CAD build for the part. Positions are in the model's coordinates, mm. Give positions to 0.01 mm unless a question says otherwise; leave off trailing zeros. Order: outer loops, then holes, each group sorted by start corner. A loop starts at its lowest first (then second) coordinate and runs counter-clockwise, first axis right, second up. Notation, with made-up numbers: (73.5, 21.25) -> (111.5, 21.25) arc R28 cw to (111.5, 45.25) -> close; hole circle Ø9 at (-14.5, 0). An arc over 180 degrees is marked (long way). Use one line per item in the form item = value. Start each with the question number.
1) Mould opens along Y. For faces 1 (the face through (0, 14, 0)), 2 (the face through (3.53, 55.87, 0.25)), 3 (the face through (-0.47, 0.67, 0.25)) say: pulls with the +Y half, pulls with the -Y half, needs draft (parallel to the pull), parting line crosses it, or undercut.
2) Cut at D-D, the plane x = -12. Give the cut face in (y, z).
3) Probe line 1 (X direction, y = 3, z = 0.4); line 2 (Y direction, x = 1, z = 0.15); line 3 (Y direction, x = 8, z = 0.4). List the from-to ranges inside material, lowest first.
4) Drop a flat-ended pin along its axis: P1, Ø3, axis at x = 7, y = -23.5, coming from the +Z side. Give the stop position or say it passes through.
5) Cut at C-C, the plane y = -21. Give the cut face in (x, z).
6) Cut at A-A, the plane x = 4. Give the cut face in (y, z), and give its area (3 significant figures).
7) Cut at B-B, the plane z = 0.35. Give the cut face in (x, y).
Autodesk Inventor part; units mm, degrees
ref_plane "YZ Plane" through (0, 0, 0) normal (1, 0, 0) x (0, 1, 0)
ref_plane "XZ Plane" through (0, 0, 0) normal (0, 1, 0) x (-1, 0, 0)
ref_plane "XY Plane" through (0, 0, 0) normal (0, 0, 1) x (1, 0, 0)
sketch "Sketch1" plane through (0, 0, 0) normal (0, 0, 1) x (1, 0, 0)
  line L0 (-17.5, -33.2499) -> (-17.5, 57.9837)
  arc A0 (-10.0449, 58.8745) -> (-17.5, 57.9837) centre (-12.5, 47.7794) ccw
  line L1 (-10.0449, 58.8745) -> (17.5, 52.7794)
  line L2 (17.5, 52.7794) -> (17.5, -15.7501)
  line L3 (17.5, -15.7501) -> (-17.5, -33.2499)
  line L4 (0.5, 7.1892) -> (0.5, 22.231)
  line L5 (0.5, 22.231) -> (-5.8925, 22.231)
  line L6 (-5.8925, 22.231) -> (-5.8925, 7.1892)
  line L7 (-5.8925, 7.1892) -> (0.5, 7.1892)
  point P0 (0, 0)
extrude "Extrusion1" add sketch "Sketch1" along normal blind 0.5 contours L0 A0 L1 L2 L3 | L7 L6 L5 L4
sketch "Sketch2" plane through (0, 0, 0.5) normal (0, 0, 1) x (1, 0, 0)
  line L0 (-1.5084, -24.1362) -> (-5.5333, -16.0863)
  line L1 (-5.5333, -16.0863) -> (-14.5107, -20.575)
  line L2 (-14.5107, -20.575) -> (-10.1014, -29.3938)
  arc A0 (-17.5, -30.0139) -> (-14.6056, -31.8027) centre (-15.5, -30.0139) ccw
  line L3 (-17.5, -30.0139) -> (-17.5, -1.8864)
  line L4 (-17.5, -1.8864) -> (-7.5, -1.8864)
  line L5 (-7.5, -1.8864) -> (-7.5, 7.5751)
  line L6 (-7.5, 7.5751) -> (-8.8, 7.5751)
  line L7 (-8.8, 26.3195) -> (-8.8, 7.5751)
  spline S0 degree 3 poles (-14.2046, 28.2052) (-13.4118, 28.2052) (-12.6544, 28.0226) (-10.9379, 27.4679) (-9.855, 26.8958) (-8.8077, 26.3237) (-8.8038, 26.3216) (-8.8, 26.3195) knots -0.001308 -0.001308 -0.001308 -0.001308 0.187612 0.187612 0.544343 0.544343 0.545651 0.545651 0.545651 0.545651
  line L8 (-14.2046, 28.2052) -> (-17.5, 28.2052)
  line L9 (-17.5, 28.2052) -> (-17.5, 31.9794)
  arc A1 (-17.5, 31.9794) -> (-4.376, 33.2499) centre (-12.5, 48.7499) ccw
  arc A2 (-4.376, 33.2499) -> (2.7674, 54.4137) centre (-12.5, 47.7794) ccw
  arc A3 (3.9006, 55.7887) -> (2.7674, 54.4137) centre (3.6845, 54.8123) ccw
  line L10 (3.9006, 55.7887) -> (16.7161, 52.9529)
  arc A4 (17.5, 51.9765) -> (16.7161, 52.9529) centre (16.5, 51.9765) ccw
  line L11 (-17.5, 57.9837) -> (-17.5, -33.2499)
  line L12 (-17.5, -33.2499) -> (17.5, -15.7501)
  line L13 (17.5, -15.7501) -> (17.5, 52.7794)
  line L14 (17.5, 52.7794) -> (-10.0449, 58.8745)
  arc A5 (-10.0449, 58.8745) -> (-17.5, 57.9837) centre (-12.5, 47.7794) ccw
  line L15 (5.1606, 7.0459) -> (-1.321, 3.6769)
  line L16 (4.7678, -6.2957) -> (11.3303, -6.2957)
  line L17 (11.3303, -6.2957) -> (11.3303, 7.0459)
  circle A6 centre (5.4296, 0.5354) radius 5.9007
  line L18 (5.4296, 0.5354) -> (11.3303, 0.5354)
  line L19 (11.3303, 0.5354) -> (11.3303, 6.4362)
  line L20 (11.3303, 6.4362) -> (5.4296, 6.4362)
  line L21 (5.4296, 6.4362) -> (5.4296, 0.5354)
  line L22 (11.3303, 0.5354) -> (5.4296, 0.5354)
  line L23 (5.4296, 0.5354) -> (5.4296, -5.3653)
  line L24 (5.4296, -5.3653) -> (11.3303, -5.3653)
  line L25 (11.3303, -5.3653) -> (11.3303, 0.5354)
  line L26 (17.5, 51.9765) -> (17.5, -14.6321)
  line L27 (17.5, -14.6321) -> (-1.4167, -24.7491)
  arc A7 (-1.4167, -24.7491) -> (-1.5084, -24.1362) centre (-2.4029, -24.5834) ccw
  line L28 (-10.1014, -29.3938) -> (-14.6056, -31.8027)
  point P0 (0, 0)
  point P1 (17.5, 7.0459)
  point P2 (17.5, -15.0638)
extrude "Extrusion2" cut sketch "Sketch2" against normal blind 10 contours L24 A6 L17 | A6 L20 L17 | L18 L21 A6 | A6 L23 L18 | A6 L21 L23
properties part number "pokrywa prawa" material "Aluminum 6061"
Result:
q1.face_1 = needs draft
q1.face_2 = pulls with the +Y half
q1.face_3 = undercut
q2.outline = (-30.5, 0) -> (59.13, 0) -> (59.13, 0.5) -> (-30.5, 0.5) -> close
q3.line_1 = -17.5 to 0.07, 11.33 to 17.5
q3.line_2 = -24 to -3.36, 4.43 to 56.43
q3.line_3 = -20.5 to -5.37, 6.44 to 54.88
q4.P1 = through
q5.outline = (-17.5, 0) -> (7, 0) -> (7, 0.5) -> (-17.5, 0.5) -> close
q6.outline = (-22.5, 0) -> (-5.19, 0) -> (-5.19, 0.5) -> (-22.5, 0.5) -> close; (6.26, 0) -> (55.77, 0) -> (55.77, 0.5) -> (6.26, 0.5) -> close
q6.area = 33.4 mm²
q7.outline = (-17.5, -33.25) -> (17.5, -15.75) -> (17.5, 52.78) -> (-10.04, 58.87) arc R11.36 ccw to (-17.5, 57.98) -> close; hole (5.43, -5.37) -> (11.33, -5.37) -> (11.33, 6.44) -> (5.43, 6.44) arc R5.9 ccw to start
